Check sheet for the modelled part. Datum: model origin and axes. Units: mm. A direction names the side the tool comes from. Coordinates: 2 decimals unless noted, no trailing zeros. Loops run counter-clockwise (first coordinate to the right, second up) from the corner with the lowest first, then second, coordinate; pieces in that order, holes last.
```python
from build123d import *

# Parameters (mm, degrees)
SKETCH1_W           = 36.75
SKETCH1_H           = 58
BOSS_EXTRUDE1_DEPTH = 3
SKETCH2_W           = 2
SKETCH2_H           = 10
BOSS_EXTRUDE2_DEPTH = 14.5
SKETCH3_R           = 1.35
CUT_EXTRUDE1_DEPTH  = 2
BOSS_EXTRUDE3_DEPTH = 25
SKETCH5_R           = 2.25
CUT_EXTRUDE2_DEPTH  = 3
SKETCH6_W           = 58
SKETCH6_H           = 3
BOSS_EXTRUDE4_DEPTH = 3
SKETCH7_R           = 6
CUT_EXTRUDE3_DEPTH  = 3
CUT_EXTRUDE4_DEPTH  = 3
SKETCH9_W           = 2
SKETCH9_H           = 14.5
BOSS_EXTRUDE5_DEPTH = 15.25
CUT_EXTRUDE5_DEPTH  = 80
SKETCH11_R          = 1.35
CUT_EXTRUDE6_DEPTH  = 3
FILLET1_R           = 2
SKETCH12_W          = 2.925
SKETCH12_H          = 18.65
SKETCH12_W_2        = 2.997200628
BOSS_EXTRUDE6_DEPTH = 25
CUT_EXTRUDE7_DEPTH  = 18.7
SKETCH14_W          = 18.45
SKETCH14_H          = 4
BOSS_EXTRUDE7_DEPTH = 25
CUT_EXTRUDE8_DEPTH  = 20.7


with BuildPart() as part:
    # Sketch1 → Boss-Extrude1 (new body)
    with BuildSketch(Plane(origin=(0, 0, 0), x_dir=(1, 0, 0), z_dir=(0, 1, 0))):
        Rectangle(SKETCH1_W, SKETCH1_H)
    extrude(amount=BOSS_EXTRUDE1_DEPTH)

    # Sketch2 → Boss-Extrude2 (add)
    with BuildSketch(Plane.XZ):
        with Locations((2.125, 24)):
            Rectangle(SKETCH2_W, SKETCH2_H)
        with Locations((2.125, -24)):
            Rectangle(SKETCH2_W, SKETCH2_H)
    extrude(amount=BOSS_EXTRUDE2_DEPTH)

    # Sketch3 → Cut-Extrude1 (cut)
    with BuildSketch(Plane(origin=(3.125, 0, 0), x_dir=(0, 0, -1), z_dir=(1, 0, 0))):
        with Locations((-24, -9)):
            Circle(SKETCH3_R)
        with Locations((24, -9)):
            Circle(SKETCH3_R)
    extrude(amount=-CUT_EXTRUDE1_DEPTH, mode=Mode.SUBTRACT)

    # Sketch4 → Boss-Extrude3 (add)
    with BuildSketch(Plane(origin=(0, 3, 0), x_dir=(1, 0, 0), z_dir=(0, 1, 0))):
        Polygon((12.775, 7.35), (0.075, 7.35), (0.075, -7.35), (12.775, -7.35), (15.775, -10.35), (-2.925, -10.35), (-2.925, 10.35), (15.775, 10.35), align=None)
    extrude(amount=BOSS_EXTRUDE3_DEPTH)

    # Sketch5 → Cut-Extrude2 (cut)
    with BuildSketch(Plane.ZY.offset(2.925)):
        with Locations((0, 8)):
            Circle(SKETCH5_R)
        with Locations((0, 23)):
            Circle(SKETCH5_R)
    extrude(amount=-CUT_EXTRUDE2_DEPTH, mode=Mode.SUBTRACT)

    # Sketch6 → Boss-Extrude4 (add)
    with BuildSketch(Plane.ZY.offset(18.375)):
        with Locations((0, 1.5)):
            Rectangle(SKETCH6_W, SKETCH6_H)
    extrude(amount=BOSS_EXTRUDE4_DEPTH)

    # Sketch7 → Cut-Extrude3 (cut)
    with BuildSketch(Plane(origin=(0, 3, 0), x_dir=(1, 0, 0), z_dir=(0, 1, 0))):
        with Locations((-11.375, 0)):
            Circle(SKETCH7_R)
    extrude(amount=-CUT_EXTRUDE3_DEPTH, mode=Mode.SUBTRACT)

    # Sketch8 → Cut-Extrude4 (cut)
    with BuildSketch(Plane(origin=(0, 3, 0), x_dir=(1, 0, 0), z_dir=(0, 1, 0))):
        Polygon((-21.375, 21), (-21.375, -21), (-13.875, -29), (-11.243766746, -32.586617788), (-32.637528156, -32.586617788), (-41.642373039, 35.783998083), (-13.875, 36.078995707), (-13.875, 29), align=None)
    extrude(amount=-CUT_EXTRUDE4_DEPTH, mode=Mode.SUBTRACT)

    # Sketch9 → Boss-Extrude5 (add)
    with BuildSketch(Plane(origin=(3.125, 0, 0), x_dir=(0, 0, -1), z_dir=(1, 0, 0))):
        with Locations((20, -7.25)):
            Rectangle(SKETCH9_W, SKETCH9_H)
        with Locations((28, -7.25)):
            Rectangle(SKETCH9_W, SKETCH9_H)
        with Locations((-28, -7.25)):
            Rectangle(SKETCH9_W, SKETCH9_H)
        with Locations((-20, -7.25)):
            Rectangle(SKETCH9_W, SKETCH9_H)
    extrude(amount=BOSS_EXTRUDE5_DEPTH)

    # Sketch10 → Cut-Extrude5 (cut, symmetric)
    with BuildSketch(Plane(origin=(0, 0, 27), x_dir=(-1, 0, 0), z_dir=(0, 0, -1))):
        Polygon((-18.375, 0), (-3.125, -14.5), (-3.818102744, -23.175648105), (-24.299297104, -22.135397869), (-27.68716384, 0.855740373), align=None)
    extrude(amount=CUT_EXTRUDE5_DEPTH, both=True, mode=Mode.SUBTRACT)

    # Sketch11 → Cut-Extrude6 (cut)
    with BuildSketch(Plane.XZ):
        with Locations((-7.875, 24)):
            Circle(SKETCH11_R)
        with Locations((-7.875, -24)):
            Circle(SKETCH11_R)
    extrude(amount=-CUT_EXTRUDE6_DEPTH, mode=Mode.SUBTRACT)

    # Fillet1
    fillet1_edges = [part.edges().sort_by_distance(p)[0] for p in [
        (-21.375, 1.5, 21),
        (-13.875, 1.5, 29),
        (-21.375, 1.5, -21),
        (-13.875, 1.5, -29),
        (18.375, 1.5, 29),
        (18.375, 1.5, -29),
    ]]
    fillet(fillet1_edges, radius=FILLET1_R)

    # Sketch12 → Boss-Extrude6 (add)
    with BuildSketch(Plane(origin=(0, 3, 0), x_dir=(1, 0, 0), z_dir=(0, 1, 0))):
        with Locations((-1.4625, -19.675)):
            Rectangle(SKETCH12_W, SKETCH12_H)
        with Locations((14.276399686, -19.675)):
            Rectangle(SKETCH12_W_2, SKETCH12_H)
        with Locations((-1.4625, 19.675)):
            Rectangle(SKETCH12_W, SKETCH12_H)
        with Locations((14.276399686, 19.675)):
            Rectangle(SKETCH12_W_2, SKETCH12_H)
    extrude(amount=BOSS_EXTRUDE6_DEPTH)

    # Sketch13 → Cut-Extrude7 (cut)
    with BuildSketch(Plane(origin=(15.775, 0, 0), x_dir=(0, 0, -1), z_dir=(1, 0, 0))):
        Polygon((-10.35, 28), (-29, 3), (-37.617706681, 3), (-37.617706681, 32.391457207), (-10.35, 32.391457207), align=None)
        Polygon((37.617706681, 32.391457207), (10.35, 32.391457207), (10.35, 28), (29, 3), (37.617706681, 3), align=None)
    extrude(amount=-CUT_EXTRUDE7_DEPTH, mode=Mode.SUBTRACT)

    # Sketch14 → Boss-Extrude7 (add)
    with BuildSketch(Plane(origin=(0, 3, 0), x_dir=(1, 0, 0), z_dir=(0, 1, 0))):
        with Locations((-12.15, 8.35)):
            Rectangle(SKETCH14_W, SKETCH14_H)
        with Locations((-12.15, -8.35)):
            Rectangle(SKETCH14_W, SKETCH14_H)
    extrude(amount=BOSS_EXTRUDE7_DEPTH)

    # Sketch15 → Cut-Extrude8 (cut)
    with BuildSketch(Plane.XY.offset(10.35)):
        Polygon((-2.925, 28), (-21.375, 3), (-26.960313264, 3), (-26.960313264, 29.401674183), (-2.925, 29.401674183), align=None)
    extrude(amount=-CUT_EXTRUDE8_DEPTH, mode=Mode.SUBTRACT)


solid = part.part
```
1) Section check A-A on x = -11.5. Enter the section's corners in (y, z).
Answer sheet:
outline: (0, -29) - (3, -29) - (3, -10.35) - (16.38, -10.35) - (16.38, -6.35) - (3, -6.35) - (3, -6) - (0, -6) - close; (0, 6) - (3, 6) - (3, 6.35) - (16.38, 6.35) - (16.38, 10.35) - (3, 10.35) - (3, 29) - (0, 29) - close
2) Section check B-B on z = 0. Enter the section's corners in (x, y) (3 decimals), plus the area to 3 significant figures.
Answer sheet:
outline: (-21.375, 0) - (-17.375, 0) - (-17.375, 3) - (-21.375, 3) - close; (-5.375, 0) - (18.375, 0) - (18.375, 3) - (0.075, 3) - (0.075, 5.75) - (-2.925, 5.75) - (-2.925, 3) - (-5.375, 3) - close; (-2.925, 10.25) - (0.075, 10.25) - (0.075, 20.75) - (-2.925, 20.75) - close; (-2.925, 25.25) - (0.075, 25.25) - (0.075, 28) - (-2.925, 28) - close
area: 131 mm2
3) Section check D-D on z = 24. Give the number of separate pieces and of enclosed holes in the cut face, plus the area to 3 significant figures.
Answer sheet:
separate pieces: 3
enclosed holes: 0
area: 166 mm2
4) Set-up check for faces 5 (the flat face through (12.778, 10, 16)), 6 (the flat face through (-21.375, 1, 0)), 7 (the flat face through (3.125, -7, -24)), 8 (the flat face through (14.297, 15.675, -19.544)), 9 (the flat face through (-8, 10, 6.35)): record each of +Z, -Z, +X, -X, +Y, -Y from which the full face is reachable in a straight line by a thin tool's end or side.
Answer sheet:
face 5: +Z, +Y
face 6: +Z, -Z, -X, +Y, -Y
face 7: +X, -Y
face 8: -Z, +X, -X, +Y
face 9: -X, +Y
5) Mould release check, pull along Y, two halves, no side actions. Record for faces 1 (the cylindrical face through (-13.79, 1.48, -28.84)), 2 (the cylindrical face through (2.139, -8.594, 22.712)), 3 (the flat face through (6, 3, -20)), 4 (the cylindrical face through (2.139, -8.594, -25.288)): +Y half, -Y half, draft (parallel to the pull), parting line (faces both ways), or undercut.
Answer sheet:
face 1: draft
face 2: undercut
face 3: +Y half
face 4: undercut
6) Scan lines: line 1 (Z direction, x = 7.5, y = -6); line 2 (Y direction, x = -2.1, z = 0); line 3 (Z direction, x = -7, y = 14). Record each from-to range of solid material in increasing order.
Answer sheet:
line 1: z = -29 to -27, -21 to -19, 19 to 21, 27 to 29
line 2: y = 0 to 5.75, 10.25 to 20.75, 25.25 to 28
line 3: z = -10.35 to -6.35, 6.35 to 10.35
7) Depth check by flat-ended pin: pin 1 (1.5 mm diameter, centred on x = 0.5, z = 5.5, fed in from -Y); pin 2 (5 mm diameter, centred on x = 13.5, z = 13.5, fed in from +Y); pin 3 (5.5 mm diameter, centred on y = 16, z = 19.5, fed in from -X) (3 decimals); pin 4 (4 mm diameter, centred on y = 8, z = 0, fed in from +X). Enter the tip coordinate at first touch or a pass-through.
Answer sheet:
pin 1: stops at y = 0
pin 2: stops at y = 27.13
pin 3: stops at x = -2.925
pin 4: passes through
